Geometry: final body of the model. Coordinates: model frame, mm. Give positions to 0.01 mm unless a question says otherwise; leave off trailing zeros. Write each loop counter-clockwise with the first axis right and the second up, starting at its lowest first coordinate (ties: lowest second). Pieces come first, ordered by that corner, then holes. Notation, with made-up numbers: (56.25, 86.5) -> (106.25, 86.5) arc R29 ccw to (106.25, 125.5) -> close; hole circle Ø9 at (9.5, 81.25). An arc over 180 degrees is marked (long way). Answer as a JSON object with one key per item and string values.
from build123d import *

# Parameters (mm, degrees)
ESTRUSIONE_SOTTILE1_DEPTH      = 120
ESTRUSIONE_SOTTILE1_DEPTH_BACK = 120
RACCORDO1_R                    = 5
RACCORDO2_R                    = 5
SCHIZZO8_R                     = 6
TAGLIO_ESTRUSIONE1_DEPTH       = 210.306999049
SCHIZZO7_R                     = 6
TAGLIO_ESTRUSIONE2_DEPTH       = 206.470737868


with BuildPart() as part:
    # Schizzo1 → Estrusione-Sottile1 (new, two sides: drawn at the far end of the back side and taken through both)
    with BuildSketch(Plane.XY.offset(-ESTRUSIONE_SOTTILE1_DEPTH_BACK)):
        with BuildLine():
            Line((0, 120), (27.957459223, 119.728070778))
            ThreePointArc((27.957459223, 119.728070778), (29.844687952, 119.338345184), (31.444362752, 118.263841181))
            Line((31.444362752, 118.263841181), (118.269943122, 31.43826081))
            ThreePointArc((118.269943122, 31.43826081), (119.341577126, 29.845406459), (119.734006879, 27.966155728))
            Line((119.734006879, 27.966155728), (120, 7))
            Line((120, 7), (121.999839065, 7.025371529))
            Line((121.999839065, 7.025371529), (121.733845944, 27.991527257))
            ThreePointArc((121.733845944, 27.991527257), (121.18444429, 30.622478281), (119.684156685, 32.852474373))
            Line((119.684156685, 32.852474373), (32.858576314, 119.678054743))
            ThreePointArc((32.858576314, 119.678054743), (30.619031595, 121.182360347), (27.976911374, 121.727976179))
            Line((27.976911374, 121.727976179), (0.019452151, 121.999905401))
            Line((0.019452151, 121.999905401), (0, 120))
        make_face()
    extrude(amount=ESTRUSIONE_SOTTILE1_DEPTH + ESTRUSIONE_SOTTILE1_DEPTH_BACK)

    # Raccordo1
    raccordo1_edges = [part.edges().sort_by_distance(p)[0] for p in [
        (120.999919532, 7.012685765, 120),
        (120.999919532, 7.012685765, -120),
    ]]
    fillet(raccordo1_edges, radius=RACCORDO1_R)

    # Raccordo2
    raccordo2_edges = [part.edges().sort_by_distance(p)[0] for p in [
        (0.009726076, 120.999952701, 120),
        (0.009726076, 120.999952701, -120),
    ]]
    fillet(raccordo2_edges, radius=RACCORDO2_R)

    # Schizzo8 → Taglio-Estrusione1 (cut, through all)
    with BuildSketch(Plane(origin=(122.069320837, 1.548667295, 0), x_dir=(0, 0, -1), z_dir=(0.9999195324498686, 0.012685764668954389, 0))):
        with Locations(Location((-97, 17.476179356, 0), (0, 0, 90))):
            Circle(SCHIZZO8_R)
        with Locations(Location((97, 17.476179356, 0), (0, 0, 90))):
            Circle(SCHIZZO8_R)
    extrude(amount=-TAGLIO_ESTRUSIONE1_DEPTH, mode=Mode.SUBTRACT)

    # Schizzo7 → Taglio-Estrusione2 (cut, through all)
    with BuildSketch(Plane(origin=(1.186526009, 121.988553816, 0), x_dir=(0.9999527006088332, -0.00972607552414292, 0), z_dir=(0.00972607552414292, 0.9999527006088332, 0))):
        with Locations(Location((13.832161446, -97, 0), (0, 0, 180))):
            Circle(SCHIZZO7_R)
        with Locations(Location((13.832161446, 97, 0), (0, 0, 180))):
            Circle(SCHIZZO7_R)
    extrude(amount=-TAGLIO_ESTRUSIONE2_DEPTH, mode=Mode.SUBTRACT)


solid = part.part
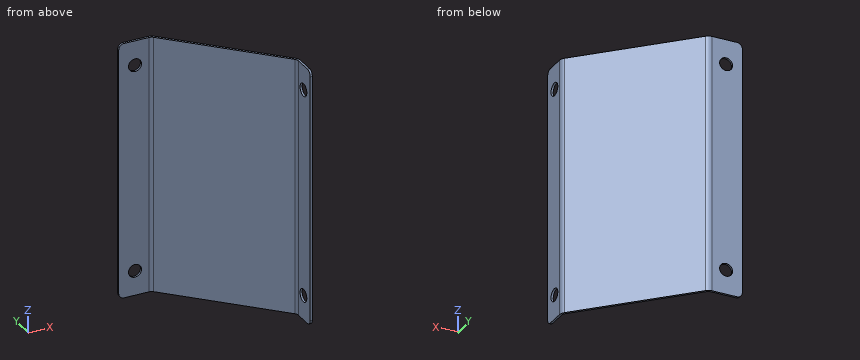
Q1. Cut plane C-C (y = 103). Return the cut outline in (x, z), and give its area (3 significant figures).
Values:
{"outline": "(46.71, -120) -> (49.54, -120) -> (49.54, 120) -> (46.71, 120) -> close", "area": "679 mm²"}
Q2. Cut plane D-D (x = 66). Return the cut outline in (y, z), and give its area (3 significant figures).
Values:
{"outline": "(83.71, -120) -> (86.54, -120) -> (86.54, 120) -> (83.71, 120) -> close", "area": "679 mm²"}
Q3. First-contact query: P1, Ø3, axis at x = 69.5, z = 55.5, coming from the -Y side; P2, Ø6, axis at y = 81.5, z = -85.5, coming from the -X side; P3, Ø6, axis at y = 108, z = -27.5, coming from the +X side; P4, Ø5, axis at x = 40, y = 104.5, coming from the +Z side. Flat tips, straight axial feed; report the tip coordinate or a pass-through.
Values:
{"P1": "y = 78.71", "P2": "x = 65.21", "P3": "x = 47.54", "P4": "through"}
Q4. Material intervals for L1, parallel to X at y = 13.5, z = 50.5; L2, parallel to Y at x = 28.5, z = -107; L3, parallel to Y at x = 6, z = 33.5, sorted ascending. Write a range as from..to.
Values:
{"L1": "119.92..121.92", "L2": "119.69..121.7", "L3": "119.94..121.94"}
Q5. Cut plane A-A (z = -58). Return the cut outline in (x, y), and give its area (3 significant figures).
Values:
{"outline": "(0, 120) -> (27.96, 119.73) arc R5 cw to (31.44, 118.26) -> (118.27, 31.44) arc R5 cw to (119.73, 27.97) -> (120, 7) -> (122, 7.03) -> (121.73, 27.99) arc R7 ccw to (119.68, 32.85) -> (32.86, 119.68) arc R7 ccw to (27.98, 121.73) -> (0.02, 122) -> close", "area": "362 mm²"}
Q6. Cut plane B-B (x = 11.5). State how many separate pieces and enclosed holes the cut face has, and give its area (3 significant figures).
Values:
{"separate pieces": "3", "enclosed holes": "0", "area": "441 mm²"}
